CAD build for the part. Positions are in the model's coordinates, mm. Face numbers are marked on the shaded views. A direction names the side the tool comes from. Coordinates: 2 decimals unless noted, no trailing zeros. Loops run counter-clockwise (first coordinate to the right, second up) from the corner with the lowest first, then second, coordinate; pieces in that order, holes last. Notation, with made-up numbers: M 86,39.25 L 133,39.25 A28 ccw 133,63.25 Z; hole C -22.5,68 d2. An arc over 180 degrees is marked long. Answer as a JSON object with one key per item and string values. Group by question number.
```python
from build123d import *

# Parameters (mm, degrees)
F0_R     = 73.9775
F1_DEPTH = 21.59
F2_DEPTH = 43.18
F3_DEPTH = 76.2
F4_DEPTH = 50.8


with BuildPart() as f1:
    # F0 (on Front) → F1 (new body)
    with BuildSketch(Plane.XZ):
        Circle(F0_R)
        with BuildLine():
            ThreePointArc((45.6497912216, 32.2284185374), (51.6263882767, 21.3843502006), (55.0682102273, 9.4903436379))
            ThreePointArc((55.0682102273, 9.4903436379), (62.3217904116, 7.0163353179), (65.405, 0))
            ThreePointArc((65.405, 0), (62.3217904116, -7.0163353179), (55.0682102273, -9.4903436379))
            ThreePointArc((55.0682102273, -9.4903436379), (51.6263882767, -21.3843502006), (45.6497912216, -32.2284185374))
            ThreePointArc((45.6497912216, -32.2284185374), (48.1496005288, -35.4960448046), (49.0381269327, -39.5131269327))
            ThreePointArc((49.0381269327, -39.5131269327), (42.7795299647, -48.4605419914), (32.2284185374, -45.6497912216))
            ThreePointArc((32.2284185374, -45.6497912216), (21.3843502006, -51.6263882767), (9.4903436379, -55.0682102273))
            ThreePointArc((9.4903436379, -55.0682102273), (9.5163319654, -55.4737354007), (9.525, -55.88))
            ThreePointArc((9.525, -55.88), (-0.4062645993, -65.3963319654), (-9.4903436379, -55.0682102273))
            ThreePointArc((-9.4903436379, -55.0682102273), (-21.3843502006, -51.6263882767), (-32.2284185374, -45.6497912216))
            ThreePointArc((-32.2284185374, -45.6497912216), (-46.2483190235, -46.2483190235), (-45.6497912216, -32.2284185374))
            ThreePointArc((-45.6497912216, -32.2284185374), (-51.6263882767, -21.3843502006), (-55.0682102273, -9.4903436379))
            ThreePointArc((-55.0682102273, -9.4903436379), (-65.405, 0), (-55.0682102273, 9.4903436379))
            ThreePointArc((-55.0682102273, 9.4903436379), (-51.6263882767, 21.3843502006), (-45.6497912216, 32.2284185374))
            ThreePointArc((-45.6497912216, 32.2284185374), (-46.2483190235, 46.2483190235), (-32.2284185374, 45.6497912216))
            ThreePointArc((-32.2284185374, 45.6497912216), (-21.3843502006, 51.6263882767), (-9.4903436379, 55.0682102273))
            ThreePointArc((-9.4903436379, 55.0682102273), (-0.4062645993, 65.3963319654), (9.525, 55.88))
            ThreePointArc((9.525, 55.88), (9.5163319654, 55.4737354007), (9.4903436379, 55.0682102273))
            ThreePointArc((9.4903436379, 55.0682102273), (21.3843502006, 51.6263882767), (32.2284185374, 45.6497912216))
            ThreePointArc((32.2284185374, 45.6497912216), (42.7795299647, 48.4605419914), (49.0381269327, 39.5131269327))
            ThreePointArc((49.0381269327, 39.5131269327), (48.1496005288, 35.4960448046), (45.6497912216, 32.2284185374))
        make_face(mode=Mode.SUBTRACT)
        with BuildLine():
            ThreePointArc((0, 38.1), (26.9407683632, 26.9407683632), (38.1, 0))
            Line((38.1, 0), (46.355, 0))
            ThreePointArc((46.355, 0), (48.8636646821, 6.4417904116), (55.0682102273, 9.4903436379))
            ThreePointArc((55.0682102273, 9.4903436379), (51.6263882767, 21.3843502006), (45.6497912216, 32.2284185374))
            ThreePointArc((45.6497912216, 32.2284185374), (32.7779348419, 32.7779348419), (32.2284185374, 45.6497912216))
            ThreePointArc((32.2284185374, 45.6497912216), (21.3843502006, 51.6263882767), (9.4903436379, 55.0682102273))
            ThreePointArc((9.4903436379, 55.0682102273), (6.4417904116, 48.8636646821), (0, 46.355))
            Line((0, 46.355), (0, 38.1))
        make_face()
        with BuildLine():
            ThreePointArc((-38.1, 0), (-26.9407683632, 26.9407683632), (0, 38.1))
            Line((0, 38.1), (0, 46.355))
            ThreePointArc((0, 46.355), (-6.4417904116, 48.8636646821), (-9.4903436379, 55.0682102273))
            ThreePointArc((-9.4903436379, 55.0682102273), (-21.3843502006, 51.6263882767), (-32.2284185374, 45.6497912216))
            ThreePointArc((-32.2284185374, 45.6497912216), (-30.565711874, 42.7795299647), (-29.9881269327, 39.5131269327))
            ThreePointArc((-29.9881269327, 39.5131269327), (-35.4960448046, 30.8766533366), (-45.6497912216, 32.2284185374))
            ThreePointArc((-45.6497912216, 32.2284185374), (-51.6263882767, 21.3843502006), (-55.0682102273, 9.4903436379))
            ThreePointArc((-55.0682102273, 9.4903436379), (-48.8636646821, 6.4417904116), (-46.355, 0))
            Line((-46.355, 0), (-38.1, 0))
        make_face()
        with BuildLine():
            Line((0, -46.355), (0, -38.1))
            ThreePointArc((0, -38.1), (-26.9407683632, -26.9407683632), (-38.1, 0))
            Line((-38.1, 0), (-46.355, 0))
            ThreePointArc((-46.355, 0), (-48.8636646821, -6.4417904116), (-55.0682102273, -9.4903436379))
            ThreePointArc((-55.0682102273, -9.4903436379), (-51.6263882767, -21.3843502006), (-45.6497912216, -32.2284185374))
            ThreePointArc((-45.6497912216, -32.2284185374), (-35.4960448046, -30.8766533366), (-29.9881269327, -39.5131269327))
            ThreePointArc((-29.9881269327, -39.5131269327), (-30.565711874, -42.7795299647), (-32.2284185374, -45.6497912216))
            ThreePointArc((-32.2284185374, -45.6497912216), (-21.3843502006, -51.6263882767), (-9.4903436379, -55.0682102273))
            ThreePointArc((-9.4903436379, -55.0682102273), (-6.4417904116, -48.8636646821), (0, -46.355))
        make_face()
        with BuildLine():
            Line((46.355, 0), (38.1, 0))
            ThreePointArc((38.1, 0), (26.9407683632, -26.9407683632), (0, -38.1))
            Line((0, -38.1), (0, -46.355))
            ThreePointArc((0, -46.355), (6.4417904116, -48.8636646821), (9.4903436379, -55.0682102273))
            ThreePointArc((9.4903436379, -55.0682102273), (21.3843502006, -51.6263882767), (32.2284185374, -45.6497912216))
            ThreePointArc((32.2284185374, -45.6497912216), (32.7779348419, -32.7779348419), (45.6497912216, -32.2284185374))
            ThreePointArc((45.6497912216, -32.2284185374), (51.6263882767, -21.3843502006), (55.0682102273, -9.4903436379))
            ThreePointArc((55.0682102273, -9.4903436379), (48.8636646821, -6.4417904116), (46.355, 0))
        make_face()
    extrude(amount=F1_DEPTH)

    # F0 (on Front) → F2 (join)
    with BuildSketch(Plane.XZ):
        with BuildLine():
            ThreePointArc((-22.225, 0), (-15.7154482119, 15.7154482119), (0, 22.225))
            Line((0, 22.225), (0, 38.1))
            ThreePointArc((0, 38.1), (-26.9407683632, 26.9407683632), (-38.1, 0))
            Line((-38.1, 0), (-22.225, 0))
        make_face()
        with BuildLine():
            Line((0, -38.1), (0, -22.225))
            ThreePointArc((0, -22.225), (-15.7154482119, -15.7154482119), (-22.225, 0))
            Line((-22.225, 0), (-38.1, 0))
            ThreePointArc((-38.1, 0), (-26.9407683632, -26.9407683632), (0, -38.1))
        make_face()
        with BuildLine():
            Line((38.1, 0), (22.225, 0))
            ThreePointArc((22.225, 0), (15.7154482119, -15.7154482119), (0, -22.225))
            Line((0, -22.225), (0, -38.1))
            ThreePointArc((0, -38.1), (26.9407683632, -26.9407683632), (38.1, 0))
        make_face()
        with BuildLine():
            ThreePointArc((0, 22.225), (15.7154482119, 15.7154482119), (22.225, 0))
            Line((22.225, 0), (38.1, 0))
            ThreePointArc((38.1, 0), (26.9407683632, 26.9407683632), (0, 38.1))
            Line((0, 38.1), (0, 22.225))
        make_face()
    extrude(amount=F2_DEPTH)

    # F0 (on Front) → F3 (join)
    with BuildSketch(Plane.XZ):
        with BuildLine():
            ThreePointArc((-12.7, 0), (-8.9802561211, 8.9802561211), (0, 12.7))
            Line((0, 12.7), (0, 22.225))
            ThreePointArc((0, 22.225), (-15.7154482119, 15.7154482119), (-22.225, 0))
            Line((-22.225, 0), (-12.7, 0))
        make_face()
        with BuildLine():
            ThreePointArc((0, 12.7), (8.9802561211, 8.9802561211), (12.7, 0))
            Line((12.7, 0), (22.225, 0))
            ThreePointArc((22.225, 0), (15.7154482119, 15.7154482119), (0, 22.225))
            Line((0, 22.225), (0, 12.7))
        make_face()
        with BuildLine():
            Line((22.225, 0), (12.7, 0))
            ThreePointArc((12.7, 0), (10.040231571, -7.7771299333), (3.175, -12.2967221242))
            Line((3.175, -12.2967221242), (3.175, -15.875))
            Line((3.175, -15.875), (0, -15.875))
            Line((0, -15.875), (0, -22.225))
            ThreePointArc((0, -22.225), (15.7154482119, -15.7154482119), (22.225, 0))
        make_face()
        with BuildLine():
            ThreePointArc((-3.175, -12.2967221242), (-10.040231571, -7.7771299333), (-12.7, 0))
            Line((-12.7, 0), (-22.225, 0))
            ThreePointArc((-22.225, 0), (-15.7154482119, -15.7154482119), (0, -22.225))
            Line((0, -22.225), (0, -15.875))
            Line((0, -15.875), (-3.175, -15.875))
            Line((-3.175, -15.875), (-3.175, -12.2967221242))
        make_face()
    extrude(amount=F3_DEPTH)

    # F0 (on Front) → F4 (join)
    with BuildSketch(Plane.XZ):
        with BuildLine():
            ThreePointArc((3.175, -12.2967221242), (10.040231571, -7.7771299333), (12.7, 0))
            Line((12.7, 0), (0, 0))
            Line((0, 0), (0, -9.525))
            Line((0, -9.525), (3.175, -9.525))
            Line((3.175, -9.525), (3.175, -12.2967221242))
        make_face()
        with BuildLine():
            Line((0, -9.525), (0, 0))
            Line((0, 0), (-12.7, 0))
            ThreePointArc((-12.7, 0), (-10.040231571, -7.7771299333), (-3.175, -12.2967221242))
            Line((-3.175, -12.2967221242), (-3.175, -9.525))
            Line((-3.175, -9.525), (0, -9.525))
        make_face()
        with BuildLine():
            Line((0, 0), (0, 12.7))
            ThreePointArc((0, 12.7), (-8.9802561211, 8.9802561211), (-12.7, 0))
            Line((-12.7, 0), (0, 0))
        make_face()
        with BuildLine():
            Line((0, 0), (12.7, 0))
            ThreePointArc((12.7, 0), (8.9802561211, 8.9802561211), (0, 12.7))
            Line((0, 12.7), (0, 0))
        make_face()
        with BuildLine():
            Line((0, -15.875), (0, -12.7))
            ThreePointArc((0, -12.7), (-1.6002545145, -12.5987771426), (-3.175, -12.2967221242))
            Line((-3.175, -12.2967221242), (-3.175, -15.875))
            Line((-3.175, -15.875), (0, -15.875))
        make_face()
        with BuildLine():
            ThreePointArc((0, -12.7), (1.6002545145, -12.5987771426), (3.175, -12.2967221242))
            Line((3.175, -12.2967221242), (3.175, -9.525))
            Line((3.175, -9.525), (0, -9.525))
            Line((0, -9.525), (0, -12.7))
        make_face()
        with BuildLine():
            Line((3.175, -15.875), (3.175, -12.2967221242))
            ThreePointArc((3.175, -12.2967221242), (1.6002545145, -12.5987771426), (0, -12.7))
            Line((0, -12.7), (0, -15.875))
            Line((0, -15.875), (3.175, -15.875))
        make_face()
        with BuildLine():
            ThreePointArc((-3.175, -12.2967221242), (-1.6002545145, -12.5987771426), (0, -12.7))
            Line((0, -12.7), (0, -9.525))
            Line((0, -9.525), (-3.175, -9.525))
            Line((-3.175, -9.525), (-3.175, -12.2967221242))
        make_face()
    extrude(amount=F4_DEPTH)


solid = f1.part
```
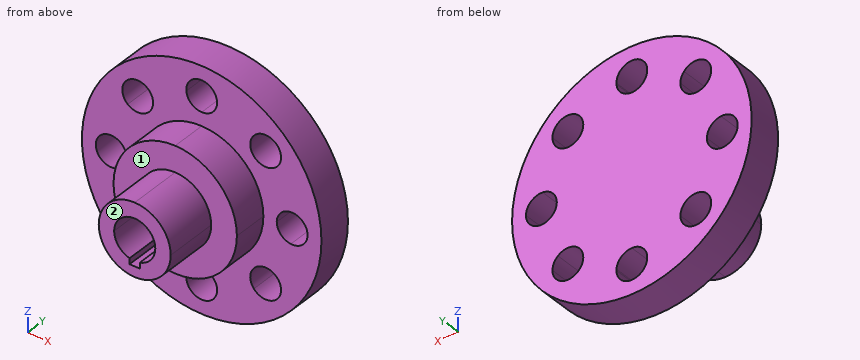
Item 1: Pin check, flat tips, straight feed: pin 1 (1 mm diameter, centred on x = -18.5, y = -27.5, fed in from -Z); pin 2 (1 mm diameter, centred on y = -39, z = 22.5, fed in from -X); pin 3 (6 mm diameter, centred on x = -25, y = -15.5, fed in from +Z); pin 4 (22 mm diameter, centred on x = -55.88, z = 0, fed in from +Y). Stop position of each tip, or through.
Item 2: Slice it at A-A, the plane y = -19. Count the separate pieces of the cut face and the enclosed holes in it, then the cut area to 3 significant figures.
Item 3: Tool access for the marked faces 1 and 2: list every direction of +Z, -Z, +X, -X, +Y, -Y with a clear straight run to the whole face (end or side of a thin tool).
Item 4: Slice it at B-B, the plane x = -43. Write the cut outline in (y, z).
Item 5: Slice it at C-C, the plane z = 58. Write the cut outline in (x, y), then the cut area to 3 significant figures.
Item 6: Slice it at D-D, the plane z = -20. Write the cut outline in (x, y), then the cut area to 3 significant figures.
Item 7: Drill centre lines: L1, parallel to X at y = -15.5, z = -0.5; L2, parallel to X at y = -15, z = -2.5; L3, parallel to Y at x = -8.5, z = -5.5. Where is each one in solid material? Low to high. Write a range as from..to.
Computed:
{
 "1": {"pin 1": "z = -33.58", "pin 2": "x = -31.11", "pin 3": "z = 70.63", "pin 4": "y = 0"},
 "2": {"separate pieces": "1", "enclosed holes": "8", "area": "14,900 mm2"},
 "3": {"face 1": "-Y", "face 2": "+Z, -Z, +X, -X, -Y"},
 "4": {"outline": "M -21.59,-60.2 L 0,-60.2 L 0,-48.38 L -21.59,-48.38 Z; M -21.59,-30.65 L 0,-30.65 L 0,30.65 L -21.59,30.65 Z; M -21.59,48.38 L 0,48.38 L 0,60.2 L -21.59,60.2 Z"},
 "5": {"outline": "M -45.92,-21.59 L -9.29,-21.59 L -9.29,0 L -45.92,0 Z; M 9.29,-21.59 L 45.92,-21.59 L 45.92,0 L 9.29,0 Z", "area": "1,580 mm2"},
 "6": {"outline": "M -71.22,-21.59 L -32.43,-21.59 L -32.43,-43.18 L -9.69,-43.18 L -9.69,-76.2 L 9.69,-76.2 L 9.69,-43.18 L 32.43,-43.18 L 32.43,-21.59 L 71.22,-21.59 L 71.22,0 L -71.22,0 Z", "area": "5,120 mm2"},
 "7": {"L1": "-73.98..-65.39, -46.37..46.37, 65.39..73.98", "L2": "-73.94..-65.07, -46.69..46.69, 65.07..73.94", "L3": "-50.8..0"}
}
